Here's how the part is built. I have some questions about the finished solid (model axes, mm). Face numbers are marked on the shaded views. A direction names the side the tool comes from. Coordinates: 2 decimals unless noted, no trailing zeros. Write each loop counter-clockwise with the first axis right and the second up, starting at its lowest first coordinate (ties: lowest second). Pieces come first, ordered by that corner, then holes. Notation, with made-up numbers: (-25.75, 76.5) -> (4.25, 76.5) arc R29 ccw to (4.25, 115.5) -> close; hole circle Ø8 at (80.25, 56). An arc over 180 degrees is marked (long way). Use CSV: the item, a comma, the result in double quotes. Start each with the question number.
```python
from build123d import *

# Parameters (mm, degrees)
SKETCH1_W           = 20
SKETCH1_H           = 80
SKETCH1_R           = 2.5
BOSS_EXTRUDE1_DEPTH = 3
SKETCH2_W           = 20
SKETCH2_H           = 3
BOSS_EXTRUDE2_DEPTH = 40
SKETCH4_W           = 3.015323491
SKETCH4_H           = 43
BOSS_EXTRUDE4_DEPTH = 20
SKETCH7_R           = 2.5
CUT_EXTRUDE2_DEPTH  = 20


with BuildPart() as part:
    # Sketch1 → Boss-Extrude1 (new body)
    with BuildSketch(Plane(origin=(0, 0, 0), x_dir=(1, 0, 0), z_dir=(0, 1, 0))):
        Rectangle(SKETCH1_W, SKETCH1_H)
        with Locations((0, -30)):
            Circle(SKETCH1_R, mode=Mode.SUBTRACT)
        with Locations((0, 10)):
            Circle(SKETCH1_R, mode=Mode.SUBTRACT)
    extrude(amount=BOSS_EXTRUDE1_DEPTH)

    # Sketch2 → Boss-Extrude2 (add)
    with BuildSketch(Plane(origin=(0, 3, 0), x_dir=(1, 0, 0), z_dir=(0, 1, 0))):
        with Locations((0, 38.5)):
            Rectangle(SKETCH2_W, SKETCH2_H)
    extrude(amount=BOSS_EXTRUDE2_DEPTH)

    # Sketch4 → Boss-Extrude4 (add)
    with BuildSketch(Plane.ZY.offset(10)):
        with Locations((-38.492338254, 21.5)):
            Rectangle(SKETCH4_W, SKETCH4_H)
    extrude(amount=BOSS_EXTRUDE4_DEPTH)

    # Sketch7 → Cut-Extrude2 (cut)
    with BuildSketch(Plane(origin=(0, 0, -40), x_dir=(-1, 0, 0), z_dir=(0, 0, -1))):
        with Locations((16, 10)):
            Circle(SKETCH7_R)
    extrude(amount=-CUT_EXTRUDE2_DEPTH, mode=Mode.SUBTRACT)


solid = part.part
```
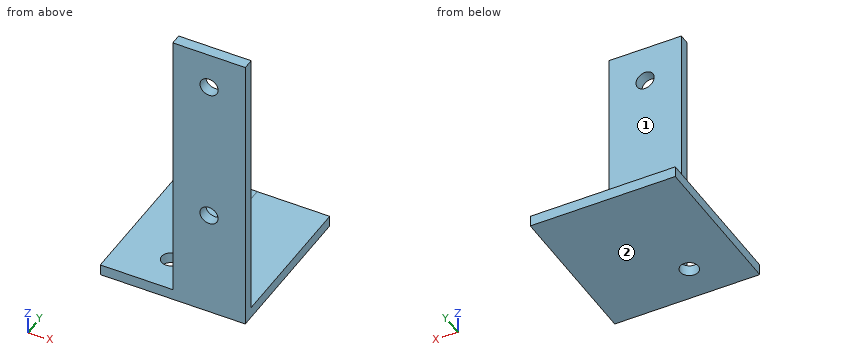
Item 1: Which directions (+Z, -Z, +X, -X, +Y, -Y) give clear straight access to the entire face, cutting with the end or side of a thin tool? Please do the marked faces 1 and 2.
Item 2: I want a section at A-A on z = -10. Please give me the cut outline in (x, y).
Item 3: I want a section at D-D on x = 0. Please give me the cut outline in (y, z).
Item 4: I want a section at B-B on x = -16. Please give me the cut outline in (y, z).
Item 5: If I drill on line 1 along Z through (x, y) = (0, 2.3); line 2 along Y through (x, z) = (-16, -39.35); line 3 along Y through (x, z) = (-4, 24), over which ranges is the centre line in solid material (lowest first)?
Item 6: I'm going to push flat-ended pins straight in: pin 1 (2.5 mm diameter, centred on y = 1.5, z = 3.5, fed in from -X); pin 2 (4 mm diameter, centred on x = 2, z = 21.5, fed in from +Y); pin 3 (10 mm diameter, centred on x = 4.5, y = 15, fed in from +Z); pin 4 (3 mm diameter, centred on x = 0, z = -10, fed in from -Y). Where does each tip first touch, or does it pass through?
Geometry says:
1,face 1,"+Z, +X, -X, +Y"
1,face 2,"-Z, +X, -X, +Y, -Y"
2,outline,"(-10, 0) -> (-2.5, 0) -> (-2.5, 3) -> (-10, 3) -> close; (2.5, 0) -> (10, 0) -> (10, 3) -> (2.5, 3) -> close"
3,outline,"(0, -40) -> (43, -40) -> (43, -37) -> (3, -37) -> (3, -12.5) -> (0, -12.5) -> close; (0, -7.5) -> (3, -7.5) -> (3, 27.5) -> (0, 27.5) -> close; (0, 32.5) -> (3, 32.5) -> (3, 40) -> (0, 40) -> close"
4,outline,"(0, -40) -> (7.5, -40) -> (7.5, -36.98) -> (0, -36.98) -> close; (12.5, -40) -> (43, -40) -> (43, -36.98) -> (12.5, -36.98) -> close"
5,line 1,"-40 to -12.5, -7.5 to 27.5, 32.5 to 40"
5,line 2,"0 to 7.5, 12.5 to 43"
5,line 3,"0 to 3"
6,pin 1,"x = -10"
6,pin 2,"y = 3"
6,pin 3,"z = -37"
6,pin 4,"through"
